```python
from build123d import *

# Parameters (mm, degrees)
ESQUISSE1_R        = 1.5
BOSS_EXTRU_1_DEPTH = 1
ESQUISSE2_W        = 13
ESQUISSE2_H        = 18
BOSS_EXTRU_2_DEPTH = 16
ESQUISSE3_W        = 16
ESQUISSE3_H        = 22
BOSS_EXTRU_3_DEPTH = 13.5
ESQUISSE4_W        = 15
ESQUISSE4_H        = 15
ESQUISSE4_H_2      = 12
BOSS_EXTRU_4_DEPTH = 7
ESQUISSE5_W        = 8.5
ESQUISSE5_H        = 7.5
BOSS_EXTRU_5_DEPTH = 3.2
CONG_3_R           = 1
CONG_4_R           = 1
ESQUISSE6_W        = 8.5
ESQUISSE6_H        = 6
BOSS_EXTRU_6_DEPTH = 3
ESQUISSE7_W        = 5
ESQUISSE7_H        = 51
BOSS_EXTRU_7_DEPTH = 8.5


with BuildPart() as part:
    # Esquisse1 → Boss.-Extru.1 (new body)
    with BuildSketch(Plane(origin=(0, 0, 0), x_dir=(1, 0, 0), z_dir=(0, 1, 0))):
        with BuildLine():
            Line((-25, -42.5), (25, -42.5))
            ThreePointArc((25, -42.5), (27.121320344, -41.621320344), (28, -39.5))
            Line((28, -39.5), (28, 39.5))
            ThreePointArc((28, 39.5), (27.121320344, 41.621320344), (25, 42.5))
            Line((25, 42.5), (-25, 42.5))
            ThreePointArc((-25, 42.5), (-27.121320344, 41.621320344), (-28, 39.5))
            Line((-28, 39.5), (-28, -39.5))
            ThreePointArc((-28, -39.5), (-27.121320344, -41.621320344), (-25, -42.5))
        make_face()
        with Locations(Location((-24.5, 39, 0), (0, 0, 270))):
            Circle(ESQUISSE1_R, mode=Mode.SUBTRACT)
        with Locations(Location((24.5, 39, 0), (0, 0, 270))):
            Circle(ESQUISSE1_R, mode=Mode.SUBTRACT)
        with Locations(Location((-24.5, -19, 0), (0, 0, 270))):
            Circle(ESQUISSE1_R, mode=Mode.SUBTRACT)
        with Locations(Location((24.5, -19, 0), (0, 0, 270))):
            Circle(ESQUISSE1_R, mode=Mode.SUBTRACT)
    extrude(amount=BOSS_EXTRU_1_DEPTH)

    # Esquisse2 → Boss.-Extru.2 (add)
    with BuildSketch(Plane(origin=(0, 1, 0), x_dir=(1, 0, 0), z_dir=(0, 1, 0))):
        with Locations((-19, -35)):
            Rectangle(ESQUISSE2_W, ESQUISSE2_H)
        with Locations((-1, -35)):
            Rectangle(ESQUISSE2_W, ESQUISSE2_H)
    extrude(amount=BOSS_EXTRU_2_DEPTH)

    # Esquisse3 → Boss.-Extru.3 (add)
    with BuildSketch(Plane(origin=(0, 1, 0), x_dir=(1, 0, 0), z_dir=(0, 1, 0))):
        with Locations((17.75, -33)):
            Rectangle(ESQUISSE3_W, ESQUISSE3_H)
    extrude(amount=BOSS_EXTRU_3_DEPTH)

    # Esquisse4 → Boss.-Extru.4 (add)
    with BuildSketch(Plane(origin=(0, 1, 0), x_dir=(1, 0, 0), z_dir=(0, 1, 0))):
        with Locations((4.5, 13.25)):
            Rectangle(ESQUISSE4_W, ESQUISSE4_H)
        with Locations((4.5, -2.25)):
            Rectangle(ESQUISSE4_W, ESQUISSE4_H_2)
    extrude(amount=BOSS_EXTRU_4_DEPTH)

    # Esquisse5 → Boss.-Extru.5 (add)
    with BuildSketch(Plane(origin=(0, 1, 0), x_dir=(1, 0, 0), z_dir=(0, 1, 0))):
        with Locations((-24.75, 31.3)):
            Rectangle(ESQUISSE5_W, ESQUISSE5_H)
    extrude(amount=BOSS_EXTRU_5_DEPTH)

    # Congé3
    cong_3_edges = [part.edges().sort_by_distance(p)[0] for p in [
        (-24.75, 4.2, -27.55),
        (-24.75, 4.2, -35.05),
    ]]
    fillet(cong_3_edges, radius=CONG_3_R)

    # Congé4
    cong_4_edges = [part.edges().sort_by_distance(p)[0] for p in [
        (-28.5, 1, -27.55),
        (-28.5, 1, -35.05),
    ]]
    fillet(cong_4_edges, radius=CONG_4_R)

    # Esquisse6 → Boss.-Extru.6 (add)
    with BuildSketch(Plane(origin=(0, 1, 0), x_dir=(1, 0, 0), z_dir=(0, 1, 0))):
        with Locations((-24.75, 16.5)):
            Rectangle(ESQUISSE6_W, ESQUISSE6_H)
        with Locations((-24.75, 3)):
            Rectangle(ESQUISSE6_W, ESQUISSE6_H)
    extrude(amount=BOSS_EXTRU_6_DEPTH)

    # Esquisse7 → Boss.-Extru.7 (add)
    with BuildSketch(Plane(origin=(0, 1, 0), x_dir=(1, 0, 0), z_dir=(0, 1, 0))):
        with Locations((24.5, 10)):
            Rectangle(ESQUISSE7_W, ESQUISSE7_H)
    extrude(amount=BOSS_EXTRU_7_DEPTH)


solid = part.part
```
Check sheet for the modelled part. Datum: model origin and axes. Units: mm. A direction names the side the tool comes from. Round coordinates to 2 decimals unless told otherwise and drop trailing zeros. Order: outer loops, then holes, each group sorted by start corner. A loop starts at its lowest first (then second) coordinate and runs counter-clockwise, first axis right, second up.
1) Go/stop test with flat-tipped pins: pin 1 Ø2 at (y, z) = (4.5, -11) entering from -X; pin 2 Ø7 at (y, z) = (6, 32.5) entering from -X; pin 3 Ø6 at (x, z) = (2.5, -32.5) entering from +Y; pin 4 Ø1.8 at (x, z) = (-24.5, 19) entering from -Y. Record where each tip stops, or that it passes through.
2) Section check D-D (z = 18.5). Record the boundary of the cut face in (x, y).
3) Scan lines: line 1 (X direction, y = 0.2, z = -39); line 2 (X direction, y = 13.25, z = 35); line 3 (X direction, y = 7.5, z = 2.5). Record each from-to range of solid material in increasing order.
4) Section check A-A (y = 7). Record the boundary of the cut face in (x, z), and give its area (3 significant figures).
5) Section check B-B (y = 15.5). Record the boundary of the cut face in (x, z), and give its area (3 significant figures).
6) Tool access check on faces 5 (the flat face through (4, 4, 8.25)), 6 (the flat face through (-25.5, 9, 35)), 7 (the flat face through (-20.5, 3, -31)), 8 (the flat face through (4, 8, 2)). Record the directions out of +Z, -Z, +X, -X, +Y, -Y that give a thin tool (end or side, any length) a straight path to the whole face; none if there is none.
7) Section check C-C (z = 35). Record the boundary of the cut face in (x, y).
8) Mould release check, pull along Z, two halves, no side actions. Record for faces 1 (the flat face through (-25, 2, -19.5)), 2 (the cylindrical face through (-27.14, 0.49, 41.6)), 3 (the flat face through (4, 4, -3.75)), 4 (the flat face through (27, 5, -10)): +Z half, -Z half, draft (parallel to the pull), parting line (faces both ways), or undercut.
Result:
1. pin 1: stops at x = -3
1. pin 2: stops at x = -25.5
1. pin 3: stops at y = 1
1. pin 4: passes through
2. outline: (-28, 0) - (-25.91, 0) - (-25.91, 1) - (-28, 1) - close; (-23.09, 0) - (23.09, 0) - (23.09, 1) - (-23.09, 1) - close; (25.91, 0) - (28, 0) - (28, 1) - (25.91, 1) - close
3. line 1: x = -28 to -26, -23 to 23, 26 to 28
3. line 2: x = -25.5 to -12.5, -7.5 to 5.5, 9.75 to 25.75
3. line 3: x = -3 to 12, 22 to 27
4. outline: (-25.5, 26) - (-12.5, 26) - (-12.5, 44) - (-25.5, 44) - close; (-7.5, 26) - (5.5, 26) - (5.5, 44) - (-7.5, 44) - close; (-3, -20.75) - (12, -20.75) - (12, -5.75) - (-3, -5.75) - close; (-3, -3.75) - (12, -3.75) - (12, 8.25) - (-3, 8.25) - close; (9.75, 22) - (25.75, 22) - (25.75, 44) - (9.75, 44) - close; (22, -35.5) - (27, -35.5) - (27, 15.5) - (22, 15.5) - close
4. area: 1,480 mm2
5. outline: (-25.5, 26) - (-12.5, 26) - (-12.5, 44) - (-25.5, 44) - close; (-7.5, 26) - (5.5, 26) - (5.5, 44) - (-7.5, 44) - close
5. area: 468 mm2
6. face 5: -X, +Y
6. face 6: +Z, -X, +Y
6. face 7: -Z, +Y
6. face 8: -Z, -X, +Y
7. outline: (-28, 0) - (28, 0) - (28, 1) - (25.75, 1) - (25.75, 14.5) - (9.75, 14.5) - (9.75, 1) - (5.5, 1) - (5.5, 17) - (-7.5, 17) - (-7.5, 1) - (-12.5, 1) - (-12.5, 17) - (-25.5, 17) - (-25.5, 1) - (-28, 1) - close
8. face 1: undercut
8. face 2: +Z half
8. face 3: undercut
8. face 4: draft
